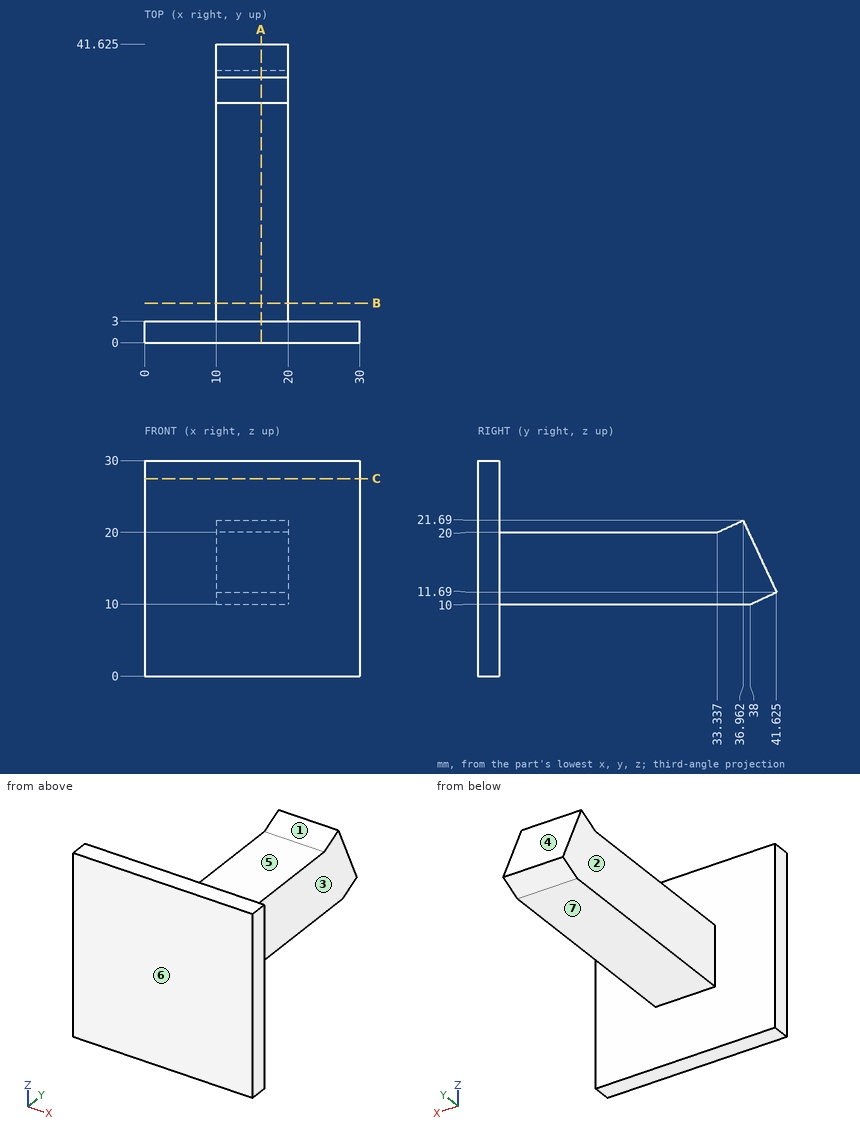
Geometry: see drawing. Coordinates: mm, zero at the bounding-box minimum. A direction names the side the tool comes from. Round coordinates to 2 decimals unless told otherwise and drop trailing zeros. Loops run counter-clockwise (first coordinate to the right, second up) from the corner with the lowest first, then second, coordinate; pieces in that order, holes last. Notation, with made-up numbers: M -28.75,8.25 L 6.25,8.25 A15 cw 6.25,26.25 Z; hole C 37.25,58.25 d6. An arc over 180 degrees is marked long. Use a Markdown table: item, result. Add a question column.
1. Cut plane B-B, the plane y = 5.5. Output: boundary loops of the cut face in (x, z), and give its area (3 significant figures).
2. Pull-direction query (Y, two-part tool) for the marked faces 5, 6 and 7; classes: +Y half, -Y half, draft (parallel to the pull), parting line (faces both ways), or undercut.
3. Contact query for flat-ended pins moving along their axis: pin 1 (8 mm diameter, centred on y = 16, z = 23, fed in from -X); pin 2 (8 mm diameter, centred on x = 14, y = 30.5, fed in from +Z); pin 3 (6 mm diameter, centred on y = 30, z = 17.5, fed in from +X). Output: stop coordinate, or through.
4. Ray query, line 1 along Z through (x, y) = (18, 8); line 2 along Y through (x, z) = (16.75, 1.5). Return the intervals inside material, ascending. Write a range as [from, to].
5. Cut plane A-A, the plane x = 16.25. Output: boundary loops of the cut face in (y, z) (1 decimal), and give its area (3 significant figures).
6. Cut plane C-C, the plane z = 27.5. Output: boundary loops of the cut face in (x, y).
7. Set-up query: the marked faces 1, 2, 3 and 4. Return all of +Z, -Z, +X, -X, +Y, -Y with unobstructed straight access to the full face (end or side cutting, diameter ignored); none if empty.
Solution:
| question | item | result |
|---|---|---|
| 1 | outline | M 10,10 L 20,10 L 20,20 L 10,20 Z |
| 1 | area | 100 mm2 |
| 2 | face 5 | undercut |
| 2 | face 6 | -Y half |
| 2 | face 7 | draft |
| 3 | pin 1 | stops at x = 10 |
| 3 | pin 2 | stops at z = 20.54 |
| 3 | pin 3 | stops at x = 20 |
| 4 | line 1 | z = [10, 20] |
| 4 | line 2 | y = [0, 3] |
| 5 | outline | M 0,0 L 3,0 L 3,10 L 38,10 L 41.6,11.7 L 37,21.7 L 33.3,20 L 3,20 L 3,30 L 0,30 Z |
| 5 | area | 461 mm2 |
| 6 | outline | M 0,0 L 30,0 L 30,3 L 0,3 Z |
| 7 | face 1 | +Z, +X, -X |
| 7 | face 2 | +Z, -Z, -X, +Y |
| 7 | face 3 | +Z, -Z, +X, +Y |
| 7 | face 4 | +Z, +X, -X, +Y |
